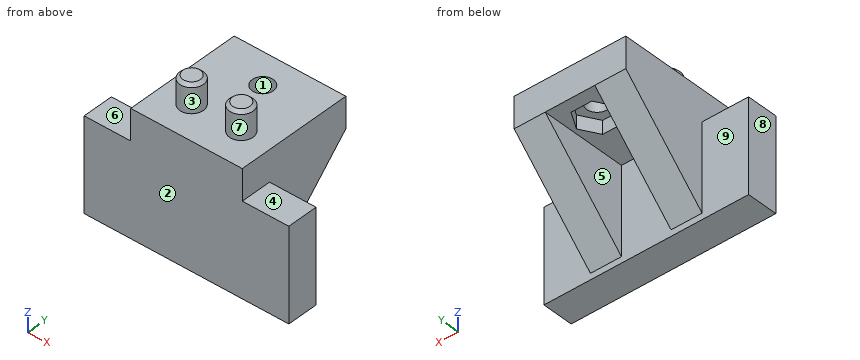
from build123d import *

# Parameters (mm, degrees)
SKETCH_W     = 18
SKETCH_H     = 19
PAD_DEPTH    = 5
SKETCH001_R  = 1.7
HOLE_DEPTH   = 5.001
POCKET_DEPTH = 2.15
SKETCH003_R  = 1.9
PAD001_DEPTH = 4.5
CHAMFER_SIZE = 0.5
SKETCH004_W  = 33
SKETCH004_H  = 5
PAD002_DEPTH = 15
PAD003_DEPTH = 5


with BuildPart() as part:
    # Sketch → Pad (new body)
    with BuildSketch(Plane.XY):
        with Locations((0, 0.5)):
            Rectangle(SKETCH_W, SKETCH_H)
    extrude(amount=PAD_DEPTH)

    # Sketch001 (on Face6 of Pad) → Hole (cut, through all)
    with BuildSketch(Plane.XY.offset(5)):
        with Locations((0, 5)):
            Circle(SKETCH001_R)
    extrude(amount=-HOLE_DEPTH, mode=Mode.SUBTRACT)

    # Sketch002 (on Face4 of Hole) → Pocket (cut)
    with BuildSketch(Plane(origin=(0, 0, 0), x_dir=(1, 0, 0), z_dir=(0, 0, -1))):
        Polygon((3.348632, -5), (1.674316, -2.1), (-1.674316, -2.1), (-3.348632, -5), (-1.674316, -7.9), (1.674316, -7.9), align=None)
    extrude(amount=-POCKET_DEPTH, mode=Mode.SUBTRACT)

    # Sketch003 (on Face5 of Pocket) → Pad001 (join)
    with BuildSketch(Plane.XY.offset(5)):
        with Locations((-4, -3.5)):
            Circle(SKETCH003_R)
    pad001 = extrude(amount=PAD001_DEPTH)

    # Mirrored: Pad001 across YZ
    add(pad001.mirror(Plane.YZ))

    # Chamfer
    chamfer_edges = [part.edges().sort_by_distance(p)[0] for p in [
        (-5.9, -3.5, 9.5),
        (5.9, -3.5, 9.5),
    ]]
    chamfer(chamfer_edges, length=CHAMFER_SIZE)

    # Sketch004 (on Face4 of Pocket) → Pad002 (join)
    with BuildSketch(Plane(origin=(0, 0, 0), x_dir=(1, 0, 0), z_dir=(0, 0, -1))):
        with Locations((0, 6.5)):
            Rectangle(SKETCH004_W, SKETCH004_H)
    extrude(amount=PAD002_DEPTH)

    # Sketch005 (on Face7 of Pad002) → Pad003 (join)
    with BuildSketch(Plane.YZ.offset(9)):
        Polygon((10, 0), (-4, -14), (-4, 0), align=None)
    pad003 = extrude(amount=-PAD003_DEPTH)

    # Mirrored001: Pad003 across YZ
    add(pad003.mirror(Plane.YZ))


solid = part.part
Input: part model. Units: mm. Frame: model coordinates. Face numbers are marked on the shaded views. A direction names the side the tool comes from. Give positions to 0.01 mm unless a question says otherwise; leave off trailing zeros. Write each loop counter-clockwise with the first axis right and the second up, starting at its lowest first coordinate (ties: lowest second). Pieces come first, ordered by that corner, then holes.
Q1. Pull-direction query (X, two-part tool) for the marked faces 6, 7, 8 and 9; classes: pulls with the +X half, pulls with the -X half, needs draft (parallel to the pull), parting line crosses it, or undercut.
Q2. Section C-C, the plane z = 4.25. Output: boundary loops of the cut face in (x, y), plus the area to 3 significant figures.
Q3. First-contact query: P1, Ø2, axis at x = 6, y = 1.5, coming from the +Z side; P2, Ø4, axis at x = -4, y = 6, coming from the -Z side; P3, Ø2.5, axis at x = 14, y = -6.5, coming from the +Z side; P4, Ø9.5, axis at y = -3, z = -2.5, coming from the -X side. Flat tips, straight axial feed; report the tip coordinate or a pass-through.
Q4. Set-up query: the marked faces 1, 2, 3, 4 and 5. Return all of +Z, -Z, +X, -X, +Y, -Y with unobstructed straight access to the full face (end or side cutting, diameter ignored); none if empty.
Q5. Section B-B, the plane y = -3.5. Output: boundary loops of the cut face in (x, z), plus the area to 3 significant figures.
Q6. Material intervals for probe 1 along Y at (x, z) = (0, 2.95); probe 2 along X at (y, z) = (5.25, 4.5); probe 3 along X at (y, z) = (5.5, -1.5), sorted ascending.
Q7. Section D-D, the plane y = 4. Output: boundary loops of the cut face in (x, z), plus the area to 3 significant figures.
Filled in:
1. face 6: needs draft
1. face 7: undercut
1. face 8: pulls with the -X half
1. face 9: undercut
2. outline: (-9, -9) - (9, -9) - (9, 10) - (-9, 10) - close; hole circle Ø3.4 at (0, 5)
2. area: 333 mm2
3. P1: stops at z = 5
3. P2: stops at z = -6
3. P3: stops at z = 0
3. P4: stops at x = -16.5
4. face 1: +Z, -Z
4. face 2: +Z, -Z, +X, -X, -Y
4. face 3: +Z
4. face 4: +Z, +X, +Y, -Y
4. face 5: -Z, +Y
5. outline: (-9, -13.5) - (-4, -13.5) - (-4, 0) - (4, 0) - (4, -13.5) - (9, -13.5) - (9, 5) - (5.9, 5) - (5.9, 9) - (5.4, 9.5) - (2.6, 9.5) - (2.1, 9) - (2.1, 5) - (-2.1, 5) - (-2.1, 9) - (-2.6, 9.5) - (-5.4, 9.5) - (-5.9, 9) - (-5.9, 5) - (-9, 5) - close
5. area: 259 mm2
6. probe 1: y = -9 to 3.3, 6.7 to 10
6. probe 2: x = -9 to -1.68, 1.68 to 9
6. probe 3: x = -9 to -4, 4 to 9
7. outline: (-9, -6) - (-4, -6) - (-4, 0) - (-2.77, 0) - (-2.77, 2.15) - (-1.37, 2.15) - (-1.37, 5) - (-9, 5) - close; (1.37, 2.15) - (2.77, 2.15) - (2.77, 0) - (4, 0) - (4, -6) - (9, -6) - (9, 5) - (1.37, 5) - close
7. area: 130 mm2
